Build history of the part. All positions in model axes, mm. A direction names the side the tool comes from. Give positions to 0.01 mm unless a question says otherwise; leave off trailing zeros. Order: outer loops, then holes, each group sorted by start corner. A loop starts at its lowest first (then second) coordinate and runs counter-clockwise, first axis right, second up. Notation, with made-up numbers: (30.25, -6.75) - (72.25, -6.75) arc R26 cw to (72.25, 18.25) - close; hole circle Ø6 at (76, 18). An arc over 180 degrees is marked (long way). One line per item, written item: value.
```python
from build123d import *

# Parameters (mm, degrees)
SKETCH1_W               = 16.75
SKETCH1_H               = 20
BOSS_EXTRUDE1_DEPTH     = 3
BOSS_EXTRUDE1_2_DEPTH   = 3
SKETCH2_W               = 45.5
SKETCH2_H               = 3
BOSS_EXTRUDE2_DEPTH     = 42
SKETCH3_R               = 8.75
CUT_EXTRUDE1_DEPTH      = 61.44447165
BOSS_EXTRUDE3_DEPTH     = 2
LPATTERN1_COUNT         = 2
LPATTERN1_PITCH         = 43.5
CUT_EXTRUDE2_DEPTH      = 61.44447165
BOSS_EXTRUDE4_DEPTH     = 3
CUT_EXTRUDE3_DEPTH      = 61.44447165
SKETCH10_W              = 10
SKETCH10_H              = 2.5
CUT_EXTRUDE4_DEPTH      = 2
BOSS_EXTRUDE5_REACH     = 66.609
SKETCH13_W              = 3
SKETCH13_H              = 11.133974596
CUT_EXTRUDE6_DEPTH      = 1
CHAMFER1_SIZE           = 1
BOSS_EXTRUDE6_DEPTH     = 13.25
CHAMFER2_SIZE           = 1
ENL_V_MAT_EXTRU_1_REACH = 59.971
ESQUISSE1_R             = 2.3


with BuildPart() as part:
    # Sketch1 → Boss-Extrude1 (new body)
    with BuildSketch(Plane.XY):
        with Locations((-28.224646897, 6.034741944)):
            Rectangle(SKETCH1_W, SKETCH1_H)
    extrude(amount=BOSS_EXTRUDE1_DEPTH)


with BuildPart() as body_2:
    # Sketch1 → Boss-Extrude1 2 (new body)
    with BuildSketch(Plane.XY):
        with Locations((0.525353103, 6.034741944)):
            Rectangle(SKETCH1_W, SKETCH1_H)
    extrude(amount=BOSS_EXTRUDE1_2_DEPTH)



with BuildPart() as body_3:
    # Sketch2 → Boss-Extrude2 (new body)
    with BuildSketch(Plane.XY.offset(3)):
        with Locations((-13.849646897, 14.534741944)):
            Rectangle(SKETCH2_W, SKETCH2_H)
    extrude(amount=BOSS_EXTRUDE2_DEPTH)

    # Sketch3 → Cut-Extrude1 (cut, through all)
    with BuildSketch(Plane(origin=(0, 13.034741944, 0), x_dir=(-1, 0, 0), z_dir=(0, -1, 0))):
        with Locations(Location((26.924646897, -35, 0), (0, 0, 90))):
            Circle(SKETCH3_R)
        with Locations(Location((0.774646897, -35, 0), (0, 0, 90))):
            Circle(SKETCH3_R)
    extrude(amount=-CUT_EXTRUDE1_DEPTH, mode=Mode.SUBTRACT)


with BuildPart() as body_2_1:
    add(body_2.part)

    add(body_3.part)  # Boss-Extrude3 merges body 3
    # Sketch4 → Boss-Extrude3 (add)
    with BuildSketch(Plane(origin=(8.900353103, 0, 0), x_dir=(0, 0, -1), z_dir=(1, 0, 0))):
        Polygon((-3, -3.965258056), (-24, 13.034741944), (-3, 13.034741944), align=None)
    boss_extrude3 = extrude(amount=-BOSS_EXTRUDE3_DEPTH)


with BuildPart() as part_1:
    add(part.part)

    add(body_2_1.part)  # LPattern1 merges body 2
    # LPattern1: Boss-Extrude3 ×2
    with Locations(*[(-i * LPATTERN1_PITCH, 0, 0) for i in range(1, LPATTERN1_COUNT)]):
        add(boss_extrude3)

    # Sketch5 → Cut-Extrude2 (cut, through all)
    with BuildSketch(Plane(origin=(0, 13.034741944, 0), x_dir=(-1, 0, 0), z_dir=(0, -1, 0))):
        Polygon((29.424646897, -8), (29.424646897, -25.5), (24.424646897, -25.5), (24.424646897, -8), (25.424646897, -8), (25.424646897, -24.5), (28.424646897, -24.5), (28.424646897, -8), align=None)
        Polygon((-0.725353103, -8), (-1.725353103, -8), (-1.725353103, -25.5), (3.274646897, -25.5), (3.274646897, -8), (2.274646897, -8), (2.274646897, -24.5), (-0.725353103, -24.5), align=None)
    extrude(amount=-CUT_EXTRUDE2_DEPTH, mode=Mode.SUBTRACT)

    # Sketch6 → Boss-Extrude4 (add)
    with BuildSketch(Plane(origin=(-25.424646897, 0, 0), x_dir=(0, 0, -1), z_dir=(1, 0, 0))):
        Polygon((-24.5, 13.034741944), (-26, 12.16871654), (-26, 10.66871654), (-21.5, 10.66871654), (-19.133974596, 13.034741944), align=None)
    boss_extrude4 = extrude(amount=-BOSS_EXTRUDE4_DEPTH)

    # Mirror7: Boss-Extrude4 across plane
    add(boss_extrude4.mirror(Plane(origin=(-13.849646897, 13.034741944, 8), x_dir=(0, 0, 1), z_dir=(1, 0, 0))))

    # Sketch9 → Cut-Extrude3 (cut, through all)
    with BuildSketch(Plane(origin=(0, 13.034741944, 0), x_dir=(-1, 0, 0), z_dir=(0, -1, 0))):
        with BuildLine():
            Line((16.849646897, -45), (10.849646897, -45))
            ThreePointArc((10.849646897, -45), (8.099646897, -42.25), (10.849646897, -39.5))
            Line((10.849646897, -39.5), (16.849646897, -39.5))
            ThreePointArc((16.849646897, -39.5), (19.599646897, -42.25), (16.849646897, -45))
        make_face()
    extrude(amount=-CUT_EXTRUDE3_DEPTH, mode=Mode.SUBTRACT)

    # Sketch10 → Cut-Extrude4 (cut)
    with BuildSketch(Plane(origin=(0, 13.034741944, 0), x_dir=(-1, 0, 0), z_dir=(0, -1, 0))):
        with Locations((13.849646897, -26.25)):
            Rectangle(SKETCH10_W, SKETCH10_H)
    extrude(amount=-CUT_EXTRUDE4_DEPTH, mode=Mode.SUBTRACT)

    # Boss-Extrude5: up to this face of the body (flat: up to its plane)
    boss_extrude5_end = Plane(part_1.part.faces().sort_by_distance((6.900353103, 7.368075277, 10))[0])
    # Sketch11 → Boss-Extrude5 (add, up to the picked face)
    with BuildSketch(Plane(origin=(-34.599646897, 0, 0), x_dir=(0, 0, -1), z_dir=(1, 0, 0)), mode=Mode.PRIVATE) as boss_extrude5_sk1:
        Polygon((-5.617808219, -1.846079974), (-3, -3.965258056), (-3, -0.465258056), (-4.5, -0.465258056), align=None)
    boss_extrude5_tool1 = split(extrude(boss_extrude5_sk1.sketch, amount=BOSS_EXTRUDE5_REACH, mode=Mode.PRIVATE), bisect_by=boss_extrude5_end, keep=Keep.BOTH, mode=Mode.PRIVATE)
    add(boss_extrude5_tool1.solids().sort_by(Axis((-34.599647, -1.87709, 3.964792), (1, 0, 0)))[0])

    # Sketch13 → Cut-Extrude6 (cut)
    with BuildSketch(Plane(origin=(0, 13.034741944, 0), x_dir=(-1, 0, 0), z_dir=(0, -1, 0))):
        with Locations((26.924646897, -13.566987298)):
            Rectangle(SKETCH13_W, SKETCH13_H)
        with Locations((0.774646897, -13.566987298)):
            Rectangle(SKETCH13_W, SKETCH13_H)
    extrude(amount=-CUT_EXTRUDE6_DEPTH, mode=Mode.SUBTRACT)

    # Chamfer1
    chamfer1_edges = [part_1.edges().sort_by_distance(p)[0] for p in [
        (-26.924646897, 14.034741944, 8),
        (-0.774646897, 14.034741944, 8),
    ]]
    chamfer(chamfer1_edges, length=CHAMFER1_SIZE - 0.0001)  # a hair under: the kernel refuses the full size

    # Sketch11<3> → Boss-Extrude6 (add)
    with BuildSketch(Plane(origin=(-34.599646897, 0, 0), x_dir=(0, 0, -1), z_dir=(1, 0, 0))):
        Polygon((-4.5, -0.465258056), (-3, -0.465258056), (-3, 1.38768312), align=None)
    boss_extrude6 = extrude(amount=BOSS_EXTRUDE6_DEPTH)

    # Mirror8: Boss-Extrude6 across plane
    add(boss_extrude6.mirror(Plane(origin=(-13.849646897, 13.034741944, 8), x_dir=(0, 0, 1), z_dir=(1, 0, 0))))

    # Chamfer2
    chamfer2_edges = [part_1.edges().sort_by_distance(p)[0] for p in [
        (-28.424646897, 14.534791944, 8),
        (-2.274646897, 14.534791944, 8),
        (-25.424646897, 14.534791944, 8),
        (0.725353103, 14.534791944, 8),
    ]]
    chamfer(chamfer2_edges, length=CHAMFER2_SIZE - 0.0001)  # a hair under: the kernel refuses the full size

    # Esquisse1 → Enlèv. mat.-Extru.1 (cut, up to next)
    with BuildSketch(Plane.XY.offset(3), mode=Mode.PRIVATE) as enl_v_mat_extru_1_sk1:
        with Locations((-3.849646897, 6.284741944)):
            Circle(ESQUISSE1_R)
    enl_v_mat_extru_1_tool1 = extrude(enl_v_mat_extru_1_sk1.sketch, amount=-ENL_V_MAT_EXTRU_1_REACH, mode=Mode.PRIVATE) & part_1.part
    # Esquisse1 → Enlèv. mat.-Extru.1 (cut, up to next)
    with BuildSketch(Plane.XY.offset(3), mode=Mode.PRIVATE) as enl_v_mat_extru_1_sk2:
        with Locations((-23.849646897, 6.284741944)):
            Circle(ESQUISSE1_R)
    enl_v_mat_extru_1_tool2 = extrude(enl_v_mat_extru_1_sk2.sketch, amount=-ENL_V_MAT_EXTRU_1_REACH, mode=Mode.PRIVATE) & part_1.part
    add(enl_v_mat_extru_1_tool1.solids().sort_by_distance((-3.849647, 6.284742, 3))[0], mode=Mode.SUBTRACT)
    add(enl_v_mat_extru_1_tool2.solids().sort_by_distance((-23.849647, 6.284742, 3))[0], mode=Mode.SUBTRACT)


solid = part_1.part
```
(1) Slice it at B-B, the plane x = -4. Give the cut face in (y, z).
Completed:
outline: (-3.97, 0) - (3.99, 0) - (3.99, 3) - (1.39, 3) - (-1.85, 5.62) - (-3.97, 3) - close; (8.58, 0) - (16.03, 0) - (16.03, 26.87) - (13.03, 26.87) - (13.03, 3) - (8.58, 3) - close; (13.03, 43.13) - (16.03, 43.13) - (16.03, 45) - (13.03, 45) - close
(2) Pin check, flat tips, straight feed: P1, Ø1, axis at x = -12, y = -2.5, coming from the -Z side; P2, Ø6, axis at x = -3, y = 3, coming from the +Z side; P3, Ø7, axis at x = -29, y = 4.5, coming from the +Z side. Stop position of each tip, or through.
Completed:
P1: z = 3
P2: z = 4.12
P3: z = 3.31
(3) Pull direction Y, two halves, no side cores. Call faces 6 (the face through (-14, 16.035, 17)), 7 (the face through (-14, 13.035, 19)), 8 (the face through (-27, 14.035, 14)): +Y half, -Y half, draft (parallel to the pull), parting line (faces both ways), or undercut.
Completed:
face 6: +Y half
face 7: undercut
face 8: -Y half
(4) Slice it at C-C, the plane z = 41. Give the cut face in (x, y).
Completed:
outline: (-36.6, 13.03) - (-33.29, 13.03) - (-33.29, 16.03) - (-36.6, 16.03) - close; (-20.56, 13.03) - (-19.3, 13.03) - (-19.3, 16.03) - (-20.56, 16.03) - close; (-8.4, 13.03) - (-7.14, 13.03) - (-7.14, 16.03) - (-8.4, 16.03) - close; (5.59, 13.03) - (8.9, 13.03) - (8.9, 16.03) - (5.59, 16.03) - close
(5) 3-axis set-ups, long thin cutter, end or side, ignore diameter. For faces 1 (the face through (-1, 15, 25.5)), 2 (the face through (-6.35, 0.1, 3.4)), 3 (the face through (-1, 10.669, 24)), 4 (the face through (-14, 15.035, 26)), 5 (the face through (1.725, 15, 17)): which of +Z, -Z, +X, -X, +Y, -Y reach the whole face in a straight line?
Completed:
face 1: +Y
face 2: +Z
face 3: +Z, +X, -X, -Y
face 4: -Y
face 5: +Y, -Y
(6) Drill centre lines: line 1 (X direction, y = 12.25, z = 20); line 2 (X direction, y = 14.45, z = 35); line 3 (X direction, y = 12.75, z = 24.5). Where is each one in solid material? Low to high.
Completed:
line 1: -36.6 to -34.6, -28.42 to -25.42, -2.27 to 0.73, 6.9 to 8.9
line 2: -36.6 to -35.67, -18.17 to -9.52, 7.98 to 8.9
line 3: -28.42 to -25.42, -2.27 to 0.73
(7) Slice it at A-A, the plane z = 35. Give the cut face in (x, y), and give its area (3 significant figures).
Completed:
outline: (-36.6, 13.03) - (-35.67, 13.03) - (-35.67, 16.03) - (-36.6, 16.03) - close; (-18.17, 13.03) - (-9.52, 13.03) - (-9.52, 16.03) - (-18.17, 16.03) - close; (7.98, 13.03) - (8.9, 13.03) - (8.9, 16.03) - (7.98, 16.03) - close
area: 31.5 mm²
(8) Slice it at D-D, the plane z = 10. Give the cut face in (x, y).
Completed:
outline: (-36.6, 1.7) - (-34.6, 1.7) - (-34.6, 13.03) - (-29.42, 13.03) - (-29.42, 16.03) - (-36.6, 16.03) - close; (-28.42, 14.03) - (-25.42, 14.03) - (-25.42, 16.03) - (-28.42, 16.03) - close; (-24.42, 13.03) - (-3.27, 13.03) - (-3.27, 16.03) - (-24.42, 16.03) - close; (-2.27, 14.03) - (0.73, 14.03) - (0.73, 16.03) - (-2.27, 16.03) - close; (1.73, 13.03) - (6.9, 13.03) - (6.9, 1.7) - (8.9, 1.7) - (8.9, 16.03) - (1.73, 16.03) - close
